Design review of the part built by this model. Coordinates are the model's own, in mm. Face numbers are marked on the shaded views. A direction names the side the tool comes from. Coordinates: 2 decimals unless noted, no trailing zeros. Loops run counter-clockwise (first coordinate to the right, second up) from the corner with the lowest first, then second, coordinate; pieces in that order, holes last.
from build123d import *

# Parameters (mm, degrees)
BASE_EXTRUSION_DEPTH    = 1
BOSS_EXTRU_1_DEPTH      = 2.5
ESQUISSE3_R             = 4
ESQUISSE3_R_2           = 2
BOSS_EXTRU_2_DEPTH      = 3
ESQUISSE4_R             = 2
ENL_V_MAT_EXTRU_1_DEPTH = 22.141379606


with BuildPart() as part:
    # Esquisse1 → Base-Extrusion (new, symmetric)
    with BuildSketch(Plane.XY):
        with BuildLine():
            Line((-5.614835193, 1), (-12, 1))
            Line((-12, 1), (-12, 3))
            Line((-12, 3), (-6, 3))
            Line((-6, 3), (1.239910882, 5.895964353))
            ThreePointArc((1.239910882, 5.895964353), (4.039542112, 6.569314748), (6.914978997, 6.417004201))
            Line((6.914978997, 6.417004201), (19, 4))
            Line((19, 4), (1.885164807, 4))
            Line((1.885164807, 4), (-5.614835193, 1))
        make_face()
    extrude(amount=BASE_EXTRUSION_DEPTH, both=True)

    # Esquisse2 → Boss.-Extru.1 (add, symmetric)
    with BuildSketch(Plane.XY):
        with BuildLine():
            Line((3.235852124, -2.351438077), (6.251216165, 1.555118833))
            ThreePointArc((6.251216165, 1.555118833), (8.004237079, 2.987515692), (10.209277422, 3.5))
            Line((10.209277422, 3.5), (13.070517185, 3.5))
            ThreePointArc((13.070517185, 3.5), (13.450300787, 3.425075357), (13.773174087, 3.211528832))
            Line((13.773174087, 3.211528832), (14.707886519, 2.288471168))
            ThreePointArc((14.707886519, 2.288471168), (15.030759819, 2.074924643), (15.410543421, 2))
            Line((15.410543421, 2), (17.381966011, 2))
            ThreePointArc((17.381966011, 2), (17.907697123, 2.149349192), (18.276393202, 2.552786405))
            Line((18.276393202, 2.552786405), (19, 4))
            Line((19, 4), (1.885164807, 4))
            Line((1.885164807, 4), (-5.614835193, 1))
            Line((-5.614835193, 1), (-12, 1))
            Line((-12, 1), (-12, 0))
            Line((-12, 0), (-8.52733926, 0))
            ThreePointArc((-8.52733926, 0), (-7.066630162, -0.218124957), (-5.733367907, -0.853468427))
            Line((-5.733367907, -0.853468427), (-2.879455607, -2.776460951))
            ThreePointArc((-2.879455607, -2.776460951), (0.277336853, -3.990373951), (3.235852124, -2.351438077))
        make_face()
    extrude(amount=BOSS_EXTRU_1_DEPTH, both=True)

    # Esquisse3 → Boss.-Extru.2 (add)
    with BuildSketch(Plane.XZ):
        with Locations((-14.5, 0)):
            Circle(ESQUISSE3_R)
        with Locations(Location((-14.5, 0, 0), (0, 0, 270))):
            Circle(ESQUISSE3_R_2, mode=Mode.SUBTRACT)
    extrude(amount=-BOSS_EXTRU_2_DEPTH)

    # Esquisse4 → Enl_v. mat.-Extru.1 (cut, through all)
    with BuildSketch(Plane(origin=(0, 0, -2.5), x_dir=(-1, 0, 0), z_dir=(0, 0, -1))):
        Circle(ESQUISSE4_R)
    extrude(amount=-ENL_V_MAT_EXTRU_1_DEPTH, mode=Mode.SUBTRACT)


solid = part.part
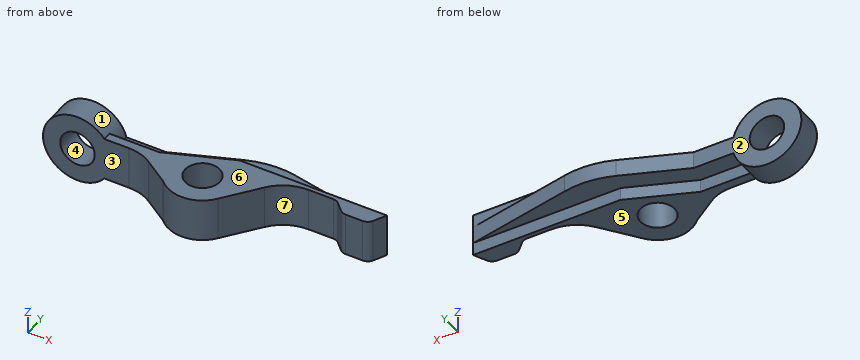
Q1. Take a section at D-D, the plane y = 5.5. Write out the cut boundary in (x, z), then the cut area to 3 significant figures.
Q2. The part is to be moulded in two halves that separate along Z. For the marked faces 4, 5, 6 and 7, say which applies: pulls with the +Z half, pulls with the -Z half, needs draft (parallel to the pull), parting line crosses it, or undercut.
Q3. For line 1 (X direction, y = 2.35, z = 0); line 2 (X direction, y = 0.7, z = 0); line 3 (Z direction, x = 3, y = 2.5), list the stretches that pass through material, from the lowest coordinate up.
Q4. Machinability: for the marked faces 1, 2 and 3, which of the approach directions +Z, -Z, +X, -X, +Y, -Y give a long, thin tool a straight path to every point of the face, cutting with its end or side? Answer none if there is none.
Q5. Take a section at B-B, the plane x = 11. Write out the cut boundary in (y, z).
Q6. Take a section at C-C, the plane x = -15. Write out the cut boundary in (y, z).
Q7. Take a section at A-A, the plane z = 0. Write out the cut boundary in (x, y).
Q8. Clearance check with flat-ended pins moving along their axes: pin 1 Ø2.5 at (x, z) = (-14.5, 0) entering from +Y; pin 2 Ø0.9 at (x, z) = (11, -1) entering from -Y; pin 3 Ø2 at (y, z) = (-1.5, 0.5) entering from -X; pin 4 Ø1.7 at (x, y) = (0.5, 5) entering from -Z. State where each tip first meets the part, or that it passes through.
Entries:
1. outline: (0.25, -1) - (11.5, -1) - (11.5, 1) - (0.25, 1) - close
1. area: 22.5 mm2
2. face 4: undercut
2. face 5: pulls with the -Z half
2. face 6: pulls with the +Z half
2. face 7: needs draft
3. line 1: x = -18.5 to -16.5, -12.5 to 7.02, 14.65 to 18.14
3. line 2: x = -18.5 to -16.5, -12.5 to -1.87, 1.87 to 5.59
3. line 3: z = -2.5 to 2.5
4. face 1: +Y
4. face 2: +Z, -Z, -X, +Y
4. face 3: +Z, -Z, -X, -Y
5. outline: (3.5, -2.5) - (4, -2.5) - (4, -1) - (5.6, -1) - (5.6, 1) - (4, 1) - (4, 2.5) - (3.5, 2.5) - close
6. outline: (0, -3.97) - (3, -3.97) - (3, -1.94) - (0, -1.94) - close; (0, 1.94) - (3, 1.94) - (3, 3.97) - (0, 3.97) - close
7. outline: (-18.5, 0) - (-16.5, 0) - (-16.5, 3) - (-18.5, 3) - close; (-12.5, 0) - (-8.53, 0) arc R5 cw to (-5.73, -0.85) - (-2.88, -2.78) arc R4 ccw to (3.24, -2.35) - (6.25, 1.56) arc R5 cw to (10.21, 3.5) - (13.07, 3.5) arc R1 cw to (13.77, 3.21) - (14.71, 2.29) arc R1 ccw to (15.41, 2) - (17.38, 2) arc R1 ccw to (18.28, 2.55) - (19, 4) - (6.91, 6.42) arc R10 ccw to (1.24, 5.9) - (-6, 3) - (-12.5, 3) - close; hole circle Ø4 at (0, 0)
8. pin 1: passes through
8. pin 2: stops at y = 3.5
8. pin 3: stops at x = -6.35
8. pin 4: stops at z = -1
